Geometry: final body of the model. Coordinates: model frame, mm. A direction names the side the tool comes from. Round coordinates to 2 decimals unless told otherwise and drop trailing zeros. Write each loop counter-clockwise with the first axis right and the second up, starting at its lowest first coordinate (ties: lowest second). Pieces come first, ordered by that corner, then holes.
from build123d import *

# Parameters (mm, degrees)
SKETCH_1_W                       = 75
SKETCH_1_H                       = 180
SM_BASE_FLANGE_1_DEPTH           = 3
SM_EDGE_FLANGE_1_STRIP_W         = 14
SM_EDGE_FLANGE_1_STRIP_H         = 3
SM_EDGE_FLANGE_1_STRIP_CUT_DEPTH = 180
SM_EDGE_FLANGE_1_DEPTH           = 180
SM_EDGE_FLANGE_2_STRIP_W         = 14
SM_EDGE_FLANGE_2_STRIP_H         = 3
SM_EDGE_FLANGE_2_STRIP_CUT_DEPTH = 180
SM_EDGE_FLANGE_2_DEPTH           = 180
CUT_EXTRUDE_12_DEPTH             = 305
CUT_EXTRUDE_13_DEPTH             = 100
SKETCH_18_R                      = 5
CUT_EXTRUDE_14_DEPTH             = 100
CUT_EXTRUDE_16_DEPTH             = 100
SKETCH_21_W                      = 73
SKETCH_21_H                      = 30
CUT_EXTRUDE_17_DEPTH             = 100
CUT_EXTRUDE_18_DEPTH             = 4
CUT_EXTRUDE_START                = -4
CUT_EXTRUDE_19_DEPTH             = 4
SKETCH_24_R                      = 4
SKETCH_24_R_2                    = 2.5
CUT_EXTRUDE_20_DEPTH             = 195.569908194
CUT_EXTRUDE_23_DEPTH             = 4
SKETCH_26_W                      = 5.11266932
SKETCH_26_H                      = 10
CUT_EXTRUDE_24_DEPTH             = 4
FILLET_1_R                       = 5
FILLET_2_R                       = 5
FILLET_3_R                       = 5
FILLET_4_R                       = 5
SKETCH_27_R                      = 3
CUT_EXTRUDE_25_DEPTH             = 202.049602951


# Read off the part's stored shape, not the designer's step: 切除-拉伸19
# Sheet-metal steps are written as plain solids
with BuildPart() as part:
    # Sketch 1 → 基体-法兰1 (new body)
    with BuildSketch(Plane.XY):
        with Locations((17.710878089, -64.466639915)):
            Rectangle(SKETCH_1_W, SKETCH_1_H)
    extrude(amount=-SM_BASE_FLANGE_1_DEPTH)

    # 边线-法兰1 strip (across the edge) → 边线-法兰1 strip cut (cut)
    with BuildSketch(Plane(origin=(55.210878089, -154.466639915, 0), x_dir=(-1, 0, 0), z_dir=(0, 1, 0))):
        with Locations((-6, -1.5)):
            Rectangle(SM_EDGE_FLANGE_1_STRIP_W, SM_EDGE_FLANGE_1_STRIP_H)
    extrude(amount=SM_EDGE_FLANGE_1_STRIP_CUT_DEPTH, mode=Mode.SUBTRACT)

    # 边线-法兰1 section (across the edge) → 边线-法兰1 (add)
    with BuildSketch(Plane(origin=(55.210878089, -154.466639915, 0), x_dir=(-1, 0, 0), z_dir=(0, 1, 0))):
        with BuildLine():
            Line((-3, 1), (-3, 100))
            Line((-3, 100), (0, 100))
            Line((0, 100), (0, 1))
            ThreePointArc((0, 1), (0.292893219, 0.292893219), (1, 0))
            Line((1, 0), (1, -3))
            ThreePointArc((1, -3), (-1.828427125, -1.828427125), (-3, 1))
        make_face()
    extrude(amount=SM_EDGE_FLANGE_1_DEPTH)

    # 边线-法兰2 strip (across the edge) → 边线-法兰2 strip cut (cut)
    with BuildSketch(Plane(origin=(-19.789121911, 25.533360085, 0), x_dir=(1, 0, 0), z_dir=(0, -1, 0))):
        with Locations((-6, -1.5)):
            Rectangle(SM_EDGE_FLANGE_2_STRIP_W, SM_EDGE_FLANGE_2_STRIP_H)
    extrude(amount=SM_EDGE_FLANGE_2_STRIP_CUT_DEPTH, mode=Mode.SUBTRACT)

    # 边线-法兰2 section (across the edge) → 边线-法兰2 (add)
    with BuildSketch(Plane(origin=(-19.789121911, 25.533360085, 0), x_dir=(1, 0, 0), z_dir=(0, -1, 0))):
        with BuildLine():
            Line((-3, 1), (-3, 100))
            Line((-3, 100), (0, 100))
            Line((0, 100), (0, 1))
            ThreePointArc((0, 1), (0.292893219, 0.292893219), (1, 0))
            Line((1, 0), (1, -3))
            ThreePointArc((1, -3), (-1.828427125, -1.828427125), (-3, 1))
        make_face()
    extrude(amount=SM_EDGE_FLANGE_2_DEPTH)

    # 草图15 → 切除-拉伸12 (cut)
    with BuildSketch(Plane(origin=(58.210878089, 0, 0), x_dir=(0, 0, -1), z_dir=(1, 0, 0))):
        Polygon((-1, -154.466639915), (-1, -134.466639915), (-90, -154.466639915), align=None)
    extrude(amount=-CUT_EXTRUDE_12_DEPTH, mode=Mode.SUBTRACT)

    # 草图17 → 切除-拉伸13 (cut)
    with BuildSketch(Plane(origin=(58.210878089, 0, 0), x_dir=(0, 0, -1), z_dir=(1, 0, 0))):
        with BuildLine():
            Line((-100, -144.217256156), (-100, -154.466639915))
            Line((-100, -154.466639915), (-90, -154.466639915))
            Line((-90, -154.466639915), (-87.840693161, -153.981343107))
            ThreePointArc((-87.840693161, -153.981343107), (-96.261267109, -152.014469389), (-100, -144.217256156))
        make_face()
    extrude(amount=-CUT_EXTRUDE_13_DEPTH, mode=Mode.SUBTRACT)

    # 草图18 → 切除-拉伸14 (cut)
    with BuildSketch(Plane(origin=(58.210878089, 0, 0), x_dir=(0, 0, -1), z_dir=(1, 0, 0))):
        with Locations((-90, -144.217256156)):
            Circle(SKETCH_18_R)
    extrude(amount=-CUT_EXTRUDE_14_DEPTH, mode=Mode.SUBTRACT)

    # 草图19 → 切除-拉伸16 (cut)
    with BuildSketch(Plane(origin=(58.210878089, 0, 0), x_dir=(0, 0, -1), z_dir=(1, 0, 0))):
        with BuildLine():
            ThreePointArc((-100, -144.217256156), (-99.436213635, -140.906988458), (-97.808425553, -137.969977518))
            Line((-97.808425553, -137.969977518), (-31, -54.466639915))
            Line((-31, -54.466639915), (-31, 25.533360085))
            Line((-31, 25.533360085), (-100, 25.533360085))
            Line((-100, 25.533360085), (-100, -144.217256156))
        make_face()
    extrude(amount=-CUT_EXTRUDE_16_DEPTH, mode=Mode.SUBTRACT)

    # 草图21 → 切除-拉伸17 (cut)
    with BuildSketch(Plane(origin=(0, 0, -3), x_dir=(-1, 0, 0), z_dir=(0, 0, -1))):
        with Locations((-17.710878089, -139.466639915)):
            Rectangle(SKETCH_21_W, SKETCH_21_H)
    extrude(amount=-CUT_EXTRUDE_17_DEPTH, mode=Mode.SUBTRACT)

    # 草图22 → 切除-拉伸18 (cut)
    with BuildSketch(Plane(origin=(0, 0, -3), x_dir=(-1, 0, 0), z_dir=(0, 0, -1))):
        Polygon((-59.141267928, -134.466639915), (-53.468887504, -134.466639915), (-53.468887504, -154.535826818), (-59.141267928, -156.162456052), align=None)
    extrude(amount=-CUT_EXTRUDE_18_DEPTH, mode=Mode.SUBTRACT)

    # 切除-拉伸19 outline → 切除-拉伸19 (cut)
    with BuildSketch(Plane(origin=(-18.789121911, 0, 0), x_dir=(0, 0, -1), z_dir=(1, 0, 0)).offset(CUT_EXTRUDE_START)):
        Polygon((3, -154.466639915), (4.115118774, -134.466639915), (-1, -134.466639915), (-1, -154.466639915), align=None)
    extrude(amount=CUT_EXTRUDE_19_DEPTH, mode=Mode.SUBTRACT)

    # 草图24 → 切除-拉伸20 (cut, through all)
    with BuildSketch(Plane(origin=(0, 0, -3), x_dir=(-1, 0, 0), z_dir=(0, 0, -1))):
        with Locations((-35.446317978, 15.533360085)):
            Circle(SKETCH_24_R)
        with Locations(Location((0.0245618, 15.533360085, 0), (0, 0, 180))):
            Circle(SKETCH_24_R)
        with Locations((-17.710878089, -39.466639915)):
            Circle(SKETCH_24_R_2)
        with Locations(Location((-17.710878089, -59.466639915, 0), (0, 0, 180))):
            Circle(SKETCH_24_R_2)
        with BuildLine():
            Line((-31.446317978, -5.021559832), (-31.446317978, -30.021559832))
            ThreePointArc((-31.446317978, -30.021559832), (-35.446317978, -34.021559832), (-39.446317978, -30.021559832))
            Line((-39.446317978, -30.021559832), (-39.446317978, -5.021559832))
            ThreePointArc((-39.446317978, -5.021559832), (-35.446317978, -1.021559832), (-31.446317978, -5.021559832))
        make_face()
        with BuildLine():
            Line((-3.9754382, -5.021559832), (-3.9754382, -30.021559832))
            ThreePointArc((-3.9754382, -30.021559832), (0.0245618, -34.021559832), (4.0245618, -30.021559832))
            Line((4.0245618, -30.021559832), (4.0245618, -5.021559832))
            ThreePointArc((4.0245618, -5.021559832), (0.0245618, -1.021559832), (-3.9754382, -5.021559832))
        make_face()
        with BuildLine():
            Line((-31.446317978, -93.911719998), (-31.446317978, -68.911719998))
            ThreePointArc((-31.446317978, -68.911719998), (-35.446317978, -64.911719998), (-39.446317978, -68.911719998))
            Line((-39.446317978, -68.911719998), (-39.446317978, -93.911719998))
            ThreePointArc((-39.446317978, -93.911719998), (-35.446317978, -97.911719998), (-31.446317978, -93.911719998))
        make_face()
        with BuildLine():
            Line((-3.9754382, -93.911719998), (-3.9754382, -68.911719998))
            ThreePointArc((-3.9754382, -68.911719998), (0.0245618, -64.911719998), (4.0245618, -68.911719998))
            Line((4.0245618, -68.911719998), (4.0245618, -93.911719998))
            ThreePointArc((4.0245618, -93.911719998), (0.0245618, -97.911719998), (-3.9754382, -93.911719998))
        make_face()
    extrude(amount=-CUT_EXTRUDE_20_DEPTH, mode=Mode.SUBTRACT)

    # 草图25 → 切除-拉伸23 (cut)
    with BuildSketch(Plane(origin=(0, 0, -3), x_dir=(-1, 0, 0), z_dir=(0, 0, -1))):
        Polygon((-54.27524735, -124.441494169), (-58.427773386, -124.441494169), (-58.210878089, -134.466639915), (-55.210878089, -134.466639915), (-54.27524735, -134.466639915), (-52.445155018, -134.466639915), (-52.445155018, -124.466639915), align=None)
    extrude(amount=-CUT_EXTRUDE_23_DEPTH, mode=Mode.SUBTRACT)

    # 草图26 → 切除-拉伸24 (cut)
    with BuildSketch(Plane(origin=(0, 0, -3), x_dir=(-1, 0, 0), z_dir=(0, 0, -1))):
        with Locations((21.345456571, -129.466639915)):
            Rectangle(SKETCH_26_W, SKETCH_26_H)
    extrude(amount=-CUT_EXTRUDE_24_DEPTH, mode=Mode.SUBTRACT)

    # 圆角1
    fillet_1_edges = [part.edges().sort_by_distance(p)[0] for p in [
        (56.710878089, -134.466639915, 1),
    ]]
    fillet(fillet_1_edges, radius=FILLET_1_R)

    # 圆角2
    fillet_2_edges = [part.edges().sort_by_distance(p)[0] for p in [
        (-21.289121911, -134.466639915, 1),
    ]]
    fillet(fillet_2_edges, radius=FILLET_2_R)

    # 圆角3
    fillet_3_edges = [part.edges().sort_by_distance(p)[0] for p in [
        (56.710878089, 25.533360085, 31),
    ]]
    fillet(fillet_3_edges, radius=FILLET_3_R)

    # 圆角4
    fillet_4_edges = [part.edges().sort_by_distance(p)[0] for p in [
        (-21.289121911, 25.533360085, 31),
    ]]
    fillet(fillet_4_edges, radius=FILLET_4_R)

    # 草图27 → 切除-拉伸25 (cut, through all)
    with BuildSketch(Plane(origin=(58.210878089, 0, 0), x_dir=(0, 0, -1), z_dir=(1, 0, 0))):
        with Locations((-6, -130.465543541)):
            Circle(SKETCH_27_R)
    extrude(amount=-CUT_EXTRUDE_25_DEPTH, mode=Mode.SUBTRACT)


solid = part.part
1) Section A-A on z = 54. Output: boundary loops of the cut face in (x, y), plus the area to 3 significant figures.
2) Draft query along X for faces 1 (the cylindrical face through (18.253, -41.907, -1.521)), 2 (the cylindrical face through (0.06, -34.02, -1.52)), 3 (the cylindrical face through (56.73, -133.13, 4.62)), 4 (the cylindrical face through (-21.586, -48.417, -1.859)). Return one class per face: pulls with the +X half, pulls with the -X half, needs draft (parallel to the pull), parting line crosses it, or undercut.
3) Section C-C on x = 9.5. Output: boundary loops of the cut face in (y, z).
4) First-contact query: P1, Ø3.5, axis at y = -23, z = -1.5, coming from the +X side; P2, Ø3.5, axis at x = 57.5, y = -20, coming from the +Z side; P3, Ø0.9, axis at y = -75.5, z = -1, coming from the -X side. Flat tips, straight axial feed; report the tip coordinate or a pass-through.
5) Section B-B on z = 75.5. Output: boundary loops of the cut face in (x, y).
6) Line query: probe 1 along X at (y, z) = (3, 22.5); probe 2 along Z at (x, y) = (-1.5, -64); probe 3 along Y at (x, z) = (57, 6). Output: solid intervals per line, ascending.
7) Reachability of faces 5 (the cylindrical face through (56.69, 24.108, 29.496)), 6 (the flat face through (-19.789, -83, 40)), 7 (the flat face through (18, 25.533, -1)), 8 (the cylindrical face through (35.534, -1.023, -1.521)) from +Z, -Z, +X, -X, +Y, -Y: full face, straight path, thin tool, end or side. Return the list, or none.
Filled in:
1. outline: (-22.79, -146.38) - (-19.79, -146.38) - (-19.79, -83.21) - (-22.79, -83.21) - close; (55.21, -146.38) - (58.21, -146.38) - (58.21, -83.21) - (55.21, -83.21) - close
1. area: 379 mm2
2. face 1: undercut
2. face 2: undercut
2. face 3: needs draft
2. face 4: pulls with the -X half
3. outline: (-124.47, -3) - (25.53, -3) - (25.53, 0) - (-124.47, 0) - close
4. P1: stops at x = 58.14
4. P2: stops at z = 31
4. P3: stops at x = -22.48
5. outline: (-22.79, -151.21) - (-19.79, -151.21) - (-19.79, -110.09) - (-22.79, -110.09) - close; (55.21, -151.21) - (58.21, -151.21) - (58.21, -110.09) - (55.21, -110.09) - close
6. probe 1: x = -22.79 to -19.79, 55.21 to 58.21
6. probe 2: z = -3 to 0
6. probe 3: y = -135.59 to -133.47, -127.47 to 25.53
7. face 5: +Z, +X, -X, +Y
7. face 6: +Z, +Y, -Y
7. face 7: +Z, -Z, +X, -X, +Y
7. face 8: +Z, -Z
